Here's how the part is built. I have some questions about the finished solid (model axes, mm). A direction names the side the tool comes from. Round coordinates to 2 decimals unless told otherwise and drop trailing zeros. Write each loop counter-clockwise with the first axis right and the second up, starting at its lowest first coordinate (ties: lowest second). Pieces come first, ordered by that corner, then holes. Notation, with made-up numbers: (16.5, 37) - (63.5, 37) arc R27 ccw to (63.5, 55) - close; hole circle Ø3 at (76, 51). An arc over 180 degrees is marked (long way). One line per item, written item: value. Start each with the question number.
Item 1: For P1, Ø1, axis at y = 7.5, z = -535.5, coming from the +X side; P2, Ø2, axis at x = 97, z = -586, coming from the -Y side; P3, Ø8, axis at x = -67.5, y = 173.5, coming from the +Z side, each with a flat end and sliding along its axis, tell me the tip position at first contact or that it passes through.
Item 2: Imagine slicing it at A-A, the plane y = 0. Please give me the cut outline in (x, z).
Item 3: Thinking about a two-plate mould opening in X: for faces 1 (the face through (-20, 46, -495)), 2 (the face through (-47.69, -15.02, -510.21)), 3 (the face through (50.453, 227.205, -499.48)), which applies, released by +X, released by -X, zero draft, split by the parting line, or undercut?
Item 4: For faces 4 (the face through (12.7, 57, -533.4)), 5 (the face through (-1, -155.5, -683.597)), which set-ups out of +Z, -Z, +X, -X, +Y, -Y let a thin tool reach every point of the face, with its end or its side?
Item 5: Imagine slicing it at C-C, the plane z = -644.5. Please give me the cut outline in (x, y), then the cut area to 3 significant figures.
Item 6: If I drill on line 1 (Y direction, x = -199.5, z = -607); line 2 (Y direction, x = 0, z = -507); line 3 (X direction, y = -127.5, z = -633), over which ranges is the centre line in solid material (lowest first)?
Item 7: Imagine slicing it at D-D, the plane z = -579. Please give me the cut outline in (x, y).
```python
from build123d import *


with BuildPart() as part:
    # Hatch Sketch → Hatch Revolution (revolve)
    with BuildSketch(Plane(origin=(0, 0, 0), x_dir=(0, 0, -1), z_dir=(1, 0, 0)), mode=Mode.PRIVATE) as hatch_revolution_sk:
        with BuildLine():
            Line((587.274308735, 273.648124971), (495, 230.651707126))
            ThreePointArc((495, 230.651707126), (518.527464888, 150), (495, 69.348292874))
            Line((495, 69.348292874), (495, 50))
            Line((495, 50), (525, 50))
            Line((525, 50), (658.847763109, 183.847763109))
            ThreePointArc((658.847763109, 183.847763109), (671.744192687, 169.975653092), (683.59650045, 155.201481952))
            Line((683.59650045, 155.201481952), (683.59650045, 208.59650045))
            ThreePointArc((683.59650045, 208.59650045), (643.910388309, 209.909991295), (606.825613004, 224.102672354))
            Line((606.825613004, 224.102672354), (621.822687178, 239.099746528))
            Line((621.822687178, 239.099746528), (587.274308735, 273.648124971))
        make_face()
    revolve(hatch_revolution_sk.sketch.rotate(Axis((0, 0, -546.1), (0, 0, 1)), 90), axis=Axis((0, 0, -546.1), (0, 0, 1)))


solid = part.part
```
Values follow:
1. P1: stops at x = 249.64
1. P2: stops at y = -255.87
1. P3: stops at z = -513.05
2. outline: (-273.65, -587.27) - (-239.1, -621.82) - (-224.1, -606.83) arc R120 cw to (-208.6, -683.6) - (-155.2, -683.6) arc R260 cw to (-183.85, -658.85) - (-50, -525) - (-50, -495) - (-69.35, -495) arc R150 cw to (-230.65, -495) - close; (50, -525) - (183.85, -658.85) arc R260 cw to (155.2, -683.6) - (208.6, -683.6) arc R120 cw to (224.1, -606.83) - (239.1, -621.82) - (273.65, -587.27) - (230.65, -495) arc R150 cw to (69.35, -495) - (50, -495) - close
3. face 1: zero draft
3. face 2: undercut
3. face 3: split by the parting line
4. face 4: none
4. face 5: -Z, +X, -X, +Y, -Y
5. outline: circle Ø419.58 at (0, 0); hole circle Ø339 at (0, 0)
5. area: 48,000 mm^2
6. line 1: y = -157.09 to -102.47, -101.86 to 101.86, 102.47 to 157.09
6. line 2: y = -236.24 to -207.67, -92.33 to -50, 50 to 92.33, 207.67 to 236.24
6. line 3: x = -170.19 to -93.32, 93.32 to 170.19
7. outline: circle Ø539.59 at (0, 0); hole circle Ø208 at (0, 0)
